from build123d import *

# Parameters (mm, degrees)
SKETCH2_R                = 2
BOSS_EXTRUDE1_DEPTH      = 17.06
SKETCH3_R                = 1.5
BOSS_EXTRUDE2_DEPTH      = 9.5
SKETCH4_W                = 3.988125856
SKETCH4_H                = 4
BOSS_EXTRUDE3_DEPTH      = 2
SKETCH5_W                = 2
SKETCH5_H                = 4
BOSS_EXTRUDE4_DEPTH      = 15
FILLET1_R                = 2
FILLET2_R                = 2
FILLET3_R                = 2
SKETCH6_R                = 1.5
CUT_EXTRUDE1_DEPTH       = 30.638380523
BOSS_EXTRUDE5_DEPTH      = 2
FILLET4_R                = 2
FILLET5_R                = 2
SKETCH8_R                = 1.5
BOSS_EXTRUDE6_DEPTH      = 36
BOSS_EXTRUDE7_DEPTH      = 1.5
BOSS_EXTRUDE7_DEPTH_BACK = 1.5
SKETCH9_R                = 2
SKETCH9_R_2              = 1.5


with BuildPart() as part:
    # Sketch2 → Boss-Extrude1 (new body)
    with BuildSketch(Plane(origin=(0, 0, 0), x_dir=(0, 0, -1), z_dir=(1, 0, 0))):
        Circle(SKETCH2_R)
    extrude(amount=BOSS_EXTRUDE1_DEPTH)

    # Sketch3 → Boss-Extrude2 (add)
    with BuildSketch(Plane(origin=(17.06, 0, 0), x_dir=(0, 0, -1), z_dir=(1, 0, 0))):
        Circle(SKETCH3_R)
    extrude(amount=BOSS_EXTRUDE2_DEPTH)

    # Sketch4 → Boss-Extrude3 (add)
    with BuildSketch(Plane(origin=(26.56, 0, 0), x_dir=(0, 0, -1), z_dir=(1, 0, 0))):
        with Locations((-0.005937072, 0)):
            Rectangle(SKETCH4_W, SKETCH4_H)
    extrude(amount=-BOSS_EXTRUDE3_DEPTH)

    # Sketch5 → Boss-Extrude4 (add)
    with BuildSketch(Plane.XY.offset(2)):
        with Locations((25.56, 0)):
            Rectangle(SKETCH5_W, SKETCH5_H)
    extrude(amount=-BOSS_EXTRUDE4_DEPTH)

    # Fillet1
    fillet1_edges = [part.edges().sort_by_distance(p)[0] for p in [
        (25.56, 2, 2),
    ]]
    fillet(fillet1_edges, radius=FILLET1_R)

    # Fillet2
    fillet2_edges = [part.edges().sort_by_distance(p)[0] for p in [
        (25.56, -2, 2),
    ]]
    fillet(fillet2_edges, radius=FILLET2_R - 0.0001)  # a hair under: the kernel refuses the full size

    # Fillet3
    fillet3_edges = [part.edges().sort_by_distance(p)[0] for p in [
        (25.56, -2, -13),
        (25.56, 2, -13),
    ]]
    fillet(fillet3_edges, radius=FILLET3_R - 0.0001)  # a hair under: the kernel refuses the full size

    # Sketch6 → Cut-Extrude1 (cut, through all)
    with BuildSketch(Plane(origin=(26.56, 0, 0), x_dir=(0, 0, -1), z_dir=(1, 0, 0))):
        with Locations((11, 0)):
            Circle(SKETCH6_R)
    extrude(amount=-CUT_EXTRUDE1_DEPTH, mode=Mode.SUBTRACT)

    # Sketch7 → Boss-Extrude5 (add)
    with BuildSketch(Plane(origin=(26.56, 0, 0), x_dir=(0, 0, -1), z_dir=(1, 0, 0))):
        with BuildLine():
            Line((18, -8.660254038), (13, 0))
            ThreePointArc((13, 0), (12.414213562, -1.414213562), (11, -2))
            Line((11, -2), (9.535898385, -2))
            Line((9.535898385, -2), (14.535898385, -10.660254038))
            Line((14.535898385, -10.660254038), (18, -8.660254038))
        make_face()
    extrude(amount=-BOSS_EXTRUDE5_DEPTH)

    # Fillet4
    fillet4_edges = [part.edges().sort_by_distance(p)[0] for p in [
        (25.56, -8.660254038, -18),
    ]]
    fillet(fillet4_edges, radius=FILLET4_R)

    # Fillet5
    fillet5_edges = [part.edges().sort_by_distance(p)[0] for p in [
        (25.56, -10.660254038, -14.535898385),
    ]]
    fillet(fillet5_edges, radius=FILLET5_R - 0.0001)  # a hair under: the kernel refuses the full size

    # Sketch8 → Boss-Extrude6 (add)
    with BuildSketch(Plane(origin=(26.56, 0, 0), x_dir=(0, 0, -1), z_dir=(1, 0, 0))):
        with Locations((15.267949192, -7.92820323)):
            Circle(SKETCH8_R)
    extrude(amount=BOSS_EXTRUDE6_DEPTH)

    # Sketch9 → Boss-Extrude7 (add, two sides: drawn at the far end of the back side and taken through both)
    # profile 1 of 4: a face of its own
    with BuildSketch(Plane(origin=(62.56, 0, 0), x_dir=(0, 0, -1), z_dir=(1, 0, 0)).offset(-BOSS_EXTRUDE7_DEPTH_BACK)):
        with Locations((15.267949192, -7.92820323)):
            Circle(SKETCH9_R)
        with Locations((15.267949192, -7.92820323)):
            Circle(SKETCH9_R_2, mode=Mode.SUBTRACT)
    # profile 2 of 4: a face of its own
    with BuildSketch(Plane(origin=(62.56, 0, 0), x_dir=(0, 0, -1), z_dir=(1, 0, 0)).offset(-BOSS_EXTRUDE7_DEPTH_BACK)):
        with BuildLine():
            ThreePointArc((13.535898385, -8.92820323), (14.267949192, -6.196152423), (17, -6.92820323))
            Line((17, -6.92820323), (13, 0))
            ThreePointArc((13, 0), (11.51763809, -1.931851653), (9.267949192, -1))
            Line((9.267949192, -1), (9.535898385, -2))
            Line((9.535898385, -2), (13.535898385, -8.92820323))
        make_face()
    # profile 3 of 4: a face of its own
    with BuildSketch(Plane(origin=(62.56, 0, 0), x_dir=(0, 0, -1), z_dir=(1, 0, 0)).offset(-BOSS_EXTRUDE7_DEPTH_BACK)):
        with BuildLine():
            ThreePointArc((9.267949192, -1), (11.51763809, -1.931851653), (13, 0))
            ThreePointArc((13, 0), (11, 2), (9, 0))
            Line((9, 0), (9.267949192, -1))
        make_face()
        with Locations((11, 0)):
            Circle(SKETCH9_R_2, mode=Mode.SUBTRACT)
    # profile 4 of 4: a face of its own
    with BuildSketch(Plane(origin=(62.56, 0, 0), x_dir=(0, 0, -1), z_dir=(1, 0, 0)).offset(-BOSS_EXTRUDE7_DEPTH_BACK)):
        with Locations((15.267949192, -7.92820323)):
            Circle(SKETCH9_R_2)
    extrude(amount=BOSS_EXTRUDE7_DEPTH + BOSS_EXTRUDE7_DEPTH_BACK)


solid = part.part
Input: part model. Units: mm. Frame: model coordinates. A direction names the side the tool comes from. Give positions to 0.01 mm unless a question says otherwise; leave off trailing zeros. Order: outer loops, then holes, each group sorted by start corner. A loop starts at its lowest first (then second) coordinate and runs counter-clockwise, first axis right, second up. Notation, with made-up numbers: (4, 74) - (35, 74) arc R30 ccw to (35, 96) - close; hole circle Ø9 at (38.5, 85). An arc over 180 degrees is marked (long way). Write each question's results on one line, items separated by ' | '.
Item 1: Material intervals for line 1 along X through (y, z) = (-2.5, -12.25); line 2 along X through (y, z) = (0.5, -2.5); line 3 along Z through (x, y) = (48, -7.75), sorted ascending.
A:
line 1: x = 24.56 to 26.56, 61.06 to 64.06 | line 2: x = 24.56 to 26.56 | line 3: z = -16.76 to -13.78
Item 2: Contact query for flat-ended pins moving along their axis: pin 1 Ø3 at (x, z) = (34, -12.5) entering from -Y; pin 2 Ø3.5 at (y, z) = (0, -11) entering from -X; pin 3 Ø8 at (x, z) = (38, -15) entering from -Y; pin 4 Ø1.8 at (y, z) = (0, -11) entering from -X. Output: stop coordinate, or through.
A:
pin 1: stops at y = -8.73 | pin 2: stops at x = 24.56 | pin 3: stops at y = -9.43 | pin 4: passes through
Item 3: Draft query along Z for faces 4 (the cylindrical face through (25.55, -1.4, 1.43)), 5 (the cylindrical face through (62.54, 0.07, -9.5)), 6 (the flat face through (61.06, -4, -13)). Return one class per face: released by +Z, released by -Z, zero draft, split by the parting line, or undercut.
A:
face 4: released by +Z | face 5: undercut | face 6: zero draft
Item 4: Section B-B (x = 11). Return loops of the section in (y, z).
A:
outline: circle Ø4 at (0, 0)
Item 5: Section A-A (y = -5). Return loops of the section in (x, z).
A:
outline: (24.56, -15.89) - (26.56, -15.89) - (26.56, -11.27) - (24.56, -11.27) - close; (61.06, -15.89) - (64.06, -15.89) - (64.06, -11.27) - (61.06, -11.27) - close
Item 6: Section D-D (x = 57.5). Return loops of the section in (y, z).
A:
outline: circle Ø3 at (-7.93, -15.27)
Item 7: Section C-C (z = -6.25). Return loops of the section in (x, y), and give its area (3 significant figures).
A:
outline: (24.56, -2) - (26.56, -2) - (26.56, 2) - (24.56, 2) - close | area: 8.00 mm^2
Item 8: Access query for faces 1 (the cylindrical face through (8, -2, 0)), 2 (the cylindrical face through (63, 2, -11)), 3 (the cylindrical face through (20.76, 0.07, 1.5)). Directions: +Z, -Z, +X, -X, +Y, -Y. A direction counts if a zero-diameter tool reaches every point of the face in a straight line with its end or side. Return the directions, or none.
A:
face 1: -X | face 2: +X, +Y | face 3: none
